```python
from build123d import *

# Parameters (mm, degrees)
SKETCH4_W           = 65
SKETCH4_H           = 30
SKETCH4_R           = 1.5
BOSS_EXTRUDE1_DEPTH = 1.8
SKETCH5_W           = 11.2
SKETCH5_H           = 7
BOSS_EXTRUDE2_DEPTH = 3.2
SKETCH6_W           = 7.4
SKETCH6_H           = 5.5
BOSS_EXTRUDE3_DEPTH = 3.3


with BuildPart() as part:
    # Sketch4 → Boss-Extrude1 (new body)
    with BuildSketch(Plane(origin=(0, 0, 0), x_dir=(1, 0, 0), z_dir=(0, 1, 0))):
        with Locations((5.223214286, 1.996173469)):
            Rectangle(SKETCH4_W, SKETCH4_H)
        with Locations((-23.776785714, 13.496173469)):
            Circle(SKETCH4_R, mode=Mode.SUBTRACT)
        with Locations((32.719505344, 13.496173469)):
            Circle(SKETCH4_R, mode=Mode.SUBTRACT)
        with Locations((34.223214286, -9.503826531)):
            Circle(SKETCH4_R, mode=Mode.SUBTRACT)
        with Locations((-23.776785714, -9.503826531)):
            Circle(SKETCH4_R, mode=Mode.SUBTRACT)
    extrude(amount=-BOSS_EXTRUDE1_DEPTH)

    # Sketch5 → Boss-Extrude2 (add)
    with BuildSketch(Plane(origin=(0, 0, 0), x_dir=(1, 0, 0), z_dir=(0, 1, 0))):
        with Locations((-14.876785714, -10.003826531)):
            Rectangle(SKETCH5_W, SKETCH5_H)
    extrude(amount=BOSS_EXTRUDE2_DEPTH)

    # Sketch6 → Boss-Extrude3 (add)
    with BuildSketch(Plane(origin=(0, 0, 0), x_dir=(1, 0, 0), z_dir=(0, 1, 0))):
        with Locations((14.123214286, -11.303826531)):
            Rectangle(SKETCH6_W, SKETCH6_H)
        with Locations((26.723214286, -11.303826531)):
            Rectangle(SKETCH6_W, SKETCH6_H)
    extrude(amount=BOSS_EXTRUDE3_DEPTH)


solid = part.part
```
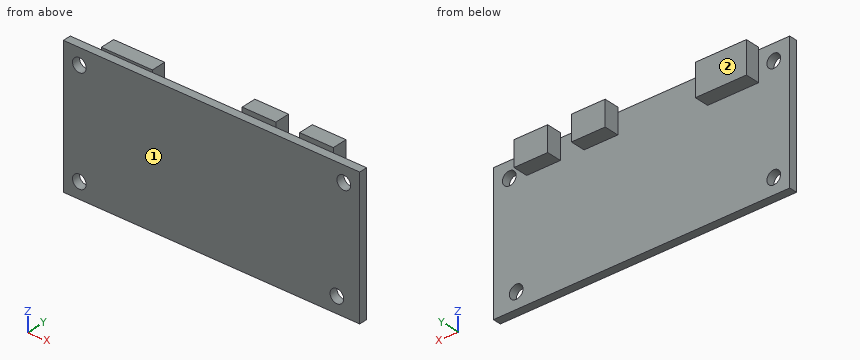
Source: CAD feature listing. Evaluate the final solid. Frame: model axes, mm. Face numbers are marked on the shaded views. A direction names the side the tool comes from. Coordinates: 2 decimals unless noted, no trailing zeros. Loops run counter-clockwise (first coordinate to the right, second up) from the corner with the lowest first, then second, coordinate; pieces in that order, holes last. Notation, with made-up numbers: M -11.75,-32 L 17.25,-32 A22 cw 17.25,-25 Z; hole C 53.25,48.25 d4. An arc over 180 degrees is marked long. Put each result on its own line as item: value. Start each with the question number.
1) Contact query for flat-ended pins moving along their axis: pin 1 Ø1 at (y, z) = (2.5, 11) entering from -X; pin 2 Ø1.6 at (x, y) = (27, 1) entering from -Z; pin 3 Ø1 at (y, z) = (1, 10) entering from +X; pin 4 Ø1.5 at (y, z) = (2, -5) entering from -X. Output: stop coordinate, or through.
2) Cut plane D-D on x = -4. Return the cut outline in (y, z), then the cut area to 3 significant figures.
3) Cut plane C-C on z = 2.5. Return the cut outline in (x, y), then the cut area to 3 significant figures.
4) Cut plane A-A on y = 1.3. Return the cut outline in (x, z), then the cut area to 3 significant figures.
5) Reachability of the marked faces 1 and 2 from +Z, -Z, +X, -X, +Y, -Y: full face, straight path, thin tool, end or side. Return the list, or none.
6) Ray query, L1, parallel to X at y = 0.45, z = 9; L2, parallel to Y at x = 15.5, z = -5; L3, parallel to Z at x = 13.5, y = -0.15. Return the intervals inside material, ascending. Write a range as from..to.
7) Cut plane B-B on x = -13. Return the cut outline in (y, z), then the cut area to 3 significant figures.
The answers:
1. pin 1: stops at x = -20.48
1. pin 2: stops at z = 8.55
1. pin 3: stops at x = 30.42
1. pin 4: passes through
2. outline: M -1.8,-17 L 0,-17 L 0,13 L -1.8,13 Z
2. area: 54.0 mm²
3. outline: M -27.28,-1.8 L 37.72,-1.8 L 37.72,0 L -27.28,0 Z
3. area: 117 mm²
4. outline: M -20.48,6.5 L -9.28,6.5 L -9.28,13.5 L -20.48,13.5 Z; M 10.42,8.55 L 17.82,8.55 L 17.82,14.05 L 10.42,14.05 Z; M 23.02,8.55 L 30.42,8.55 L 30.42,14.05 L 23.02,14.05 Z
4. area: 160 mm²
5. face 1: +Z, -Z, +X, -X, -Y
5. face 2: +Z, -Z, -X, +Y
6. L1: x = -20.48..-9.28, 10.42..17.82, 23.02..30.42
6. L2: y = -1.8..0
6. L3: z = -17..13
7. outline: M -1.8,-17 L 0,-17 L 0,6.5 L 3.2,6.5 L 3.2,13.5 L 0,13.5 L 0,13 L -1.8,13 Z
7. area: 76.4 mm²
